Can you work these out from the drawing? Everything is in mm from the part's minimum corner. A direction names the side the tool comes from. Give positions to 0.01 mm unless a question says otherwise; leave off trailing zeros. Write each loop counter-clockwise with the first axis right and the second up, starting at its lowest first coordinate (ties: lowest second). Pieces come first, ordered by that corner, then holes. Notation, with made-up numbers: (-25, -30) - (-13, -30) arc R17 cw to (-13, -1) - close; hole circle Ø9 at (-15, 0). An arc over 180 degrees is marked (long way). Use a Markdown table: item, result. Add a question column.
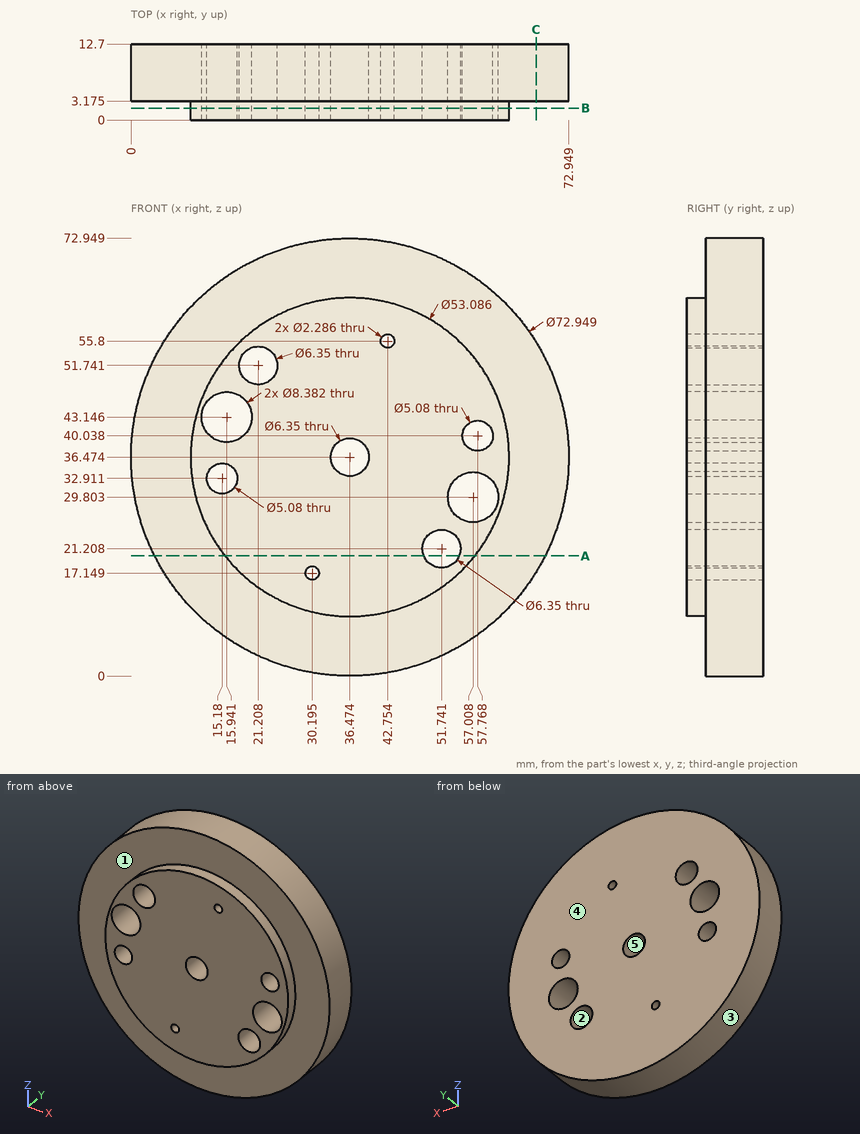
Q1. Suppose I cut it at C-C (x = 67.5). Please give me the cut outline in (y, z) (1 decimal).
Q2. Suppose I cut it at B-B (y = 2). Give the number of separate pieces and of enclosed holes in the cut face, and give its area (3 significant figures).
Q3. Suppose I cut it at A-A (z = 20). Please give me the cut outline in (x, y) (1 decimal).
Q4. I'm going to push flat-ended pins straight in: P1, Ø6, axis at x = 31, y = 8, coming from the -Z side; P2, Ø6, axis at y = 6.5, z = 33, coming from the +X side; P3, Ø5, axis at x = 11, z = 62, coming from the -Y side (1 decimal). Where does each tip first touch, or does it pass through?
Q5. On a 3-axis mill with a long thin cutter (end or side, diameter ignored), from which of +Z, -Z, +X, -X, +Y, -Y can I reach the whole of each face in a straight line? I mean the marked faces 1 and 2. Say none if no direction works.
Q6. If I drill on probe 1 along Y at (x, z) = (38, 70) (1 decimal); probe 2 along X at (y, z) = (4.75, 22.5) (1 decimal); probe 3 along Z at (x, y) = (59.5, 4.75) (1 decimal), over which ranges is the centre line in solid material (lowest first)? Write a range as [from, to].
Q7. If we mould it in two halves opening along Z, with no side actions, what happens to the marked faces 3, 4 and 5? For each: released by +Z, released by -Z, zero draft, split by the parting line, or undercut.
Derived:
| question | item | result |
|---|---|---|
| 1 | outline | (3.2, 17.3) - (12.7, 17.3) - (12.7, 55.7) - (3.2, 55.7) - close |
| 2 | separate pieces | 1 |
| 2 | enclosed holes | 9 |
| 2 | area | 1,960 mm² |
| 3 | outline | (3.9, 3.2) - (15.7, 3.2) - (15.7, 0) - (48.8, 0) - (48.8, 12.7) - (3.9, 12.7) - close; (54.7, 0) - (57.3, 0) - (57.3, 3.2) - (69, 3.2) - (69, 12.7) - (54.7, 12.7) - close |
| 4 | P1 | z = 0.08 |
| 4 | P2 | x = 72.95 |
| 4 | P3 | y = 3.2 |
| 5 | face 1 | -Y |
| 5 | face 2 | +Y, -Y |
| 6 | probe 1 | [3.2, 12.7] |
| 6 | probe 2 | [2.8, 48.8], [54.6, 70.2] |
| 6 | probe 3 | [8.2, 26.4], [33.2, 38.2], [41.9, 64.8] |
| 7 | face 3 | split by the parting line |
| 7 | face 4 | zero draft |
| 7 | face 5 | undercut |
